from build123d import *

# Parameters (mm, degrees)
SKETCH1_R           = 1.375
SKETCH1_R_2         = 1.4
BOSS_EXTRUDE1_DEPTH = 1.5


with BuildPart() as part:
    # Sketch1 → Boss-Extrude1 (new body)
    # profile 1 of 2: a face of its own
    with BuildSketch(Plane.XY):
        Polygon((37, 12), (37, 0), (-37, 0), (-37, 12), (-68.380126203, 43.380126203), (-65.551699078, 46.208553328), (-31.343145751, 12), (31.343145751, 12), (65.562445841, 46.21930009), (68.390872965, 43.390872965), align=None)
        with Locations((29, 5)):
            Circle(SKETCH1_R, mode=Mode.SUBTRACT)
        with Locations((-29, 5)):
            Circle(SKETCH1_R, mode=Mode.SUBTRACT)
    # profile 2 of 2: a face of its own
    with BuildSketch(Plane.XY):
        Polygon((-5, 46.213516444), (-65.551699078, 46.208553328), (-56.343145751, 37), (56.343145751, 37), (65.562445841, 46.21930009), (5, 46.214336093), (5, 38.213516444), (-5, 38.213516444), align=None)
        with Locations((-10.5, 41.713065622)):
            Circle(SKETCH1_R_2, mode=Mode.SUBTRACT)
        with Locations((10.499999929, 41.714786885)):
            Circle(SKETCH1_R_2, mode=Mode.SUBTRACT)
    extrude(amount=BOSS_EXTRUDE1_DEPTH)


solid = part.part
Read the model definition and answer for the solid it produces. Units are mm, in the model's axes. A direction names the side the tool comes from. Round coordinates to 2 decimals unless told otherwise and drop trailing zeros. Write each loop counter-clockwise with the first axis right and the second up, starting at its lowest first coordinate (ties: lowest second). Pieces come first, ordered by that corner, then holes.
1. Which of the six approach directions +Z, -Z, +X, -X, +Y, -Y give full straight-line access (tool end or side, diameter ignored) to faces 1 (the face through (43.668, 24.325, 0.74)), 2 (the face through (-52, 27, 1))?
2. The part is cut by section D-D, the plane y = 16.5. Determine the outline of the cut face in (x, z), then the cut area to 3 significant figures.
3. The part is cut by section C-C, the plane z = 0.8. Determine the outline of the cut face in (x, y) (3 decimals).
4. The part is cut by section A-A, the plane y = 5. Determine the outline of the cut face in (x, z) (3 decimals), then the cut area to 3 significant figures.
5. Given pin 1 Ø2.5 at (x, y) = (10.5, 41.71) entering from -Z; pin 2 Ø3.5 at (x, y) = (29, 5) entering from +Z; pin 3 Ø0.8 at (y, z) = (7, 1) entering from +X, each flat-ended and moving along its own axis, determine where each tip first touches the part or whether it passes through.
6. Straight lines are drawn through the part: L1, parallel to Y at x = 29, z = 1.15 (3 decimals); L2, parallel to Y at x = 10.5, z = 1; L3, parallel to Y at x = 15, z = 0.25. For each, find the intervals that lie inside material, in ascending order.
7. Determine the mould class of faces 3 (the face through (-5.4, 38.6, 0)), 4 (the face through (-44.018, 24.675, 0.74)), 5 (the face through (-66.99, 44.77, 0.74)) for opening direction X: pulls with the +X half, pulls with the -X half, needs draft (parallel to the pull), parting line crosses it, or undercut.
8. The part is cut by section B-B, the plane x = 10.5. Determine the outline of the cut face in (y, z).
Values:
1. face 1: +Z, -Z
1. face 2: +Z, -Z, -X, -Y
2. outline: (-41.5, 0) - (-35.84, 0) - (-35.84, 1.5) - (-41.5, 1.5) - close; (35.84, 0) - (41.5, 0) - (41.5, 1.5) - (35.84, 1.5) - close
2. area: 17.0 mm2
3. outline: (-68.38, 43.38) - (-37, 12) - (-37, 0) - (37, 0) - (37, 12) - (68.391, 43.391) - (65.562, 46.219) - (5, 46.214) - (5, 38.214) - (-5, 38.214) - (-5, 46.214) - (-65.552, 46.209) - close; hole (-56.343, 37) - (-31.343, 12) - (31.343, 12) - (56.343, 37) - close; hole circle Ø2.75 at (-29, 5); hole circle Ø2.8 at (-10.5, 41.713); hole circle Ø2.8 at (10.5, 41.715); hole circle Ø2.75 at (29, 5)
4. outline: (-37, 0) - (-30.375, 0) - (-30.375, 1.5) - (-37, 1.5) - close; (-27.625, 0) - (27.625, 0) - (27.625, 1.5) - (-27.625, 1.5) - close; (30.375, 0) - (37, 0) - (37, 1.5) - (30.375, 1.5) - close
4. area: 103 mm2
5. pin 1: passes through
5. pin 2: stops at z = 1.5
5. pin 3: stops at x = 37
6. L1: y = 0 to 3.625, 6.375 to 12, 37 to 46.216
6. L2: y = 0 to 12, 37 to 40.31, 43.11 to 46.21
6. L3: y = 0 to 12, 37 to 46.22
7. face 3: needs draft
7. face 4: undercut
7. face 5: pulls with the -X half
8. outline: (0, 0) - (12, 0) - (12, 1.5) - (0, 1.5) - close; (37, 0) - (40.31, 0) - (40.31, 1.5) - (37, 1.5) - close; (43.11, 0) - (46.21, 0) - (46.21, 1.5) - (43.11, 1.5) - close
